from build123d import *

# Parameters (mm, degrees)
F0_W     = 23
F0_H     = 10
F1_DEPTH = 4
F3_DEPTH = 10.001
F4_W     = 19
F4_H     = 6
F5_DEPTH = 8.001
F6_W     = 6
F6_H     = 4
F8_W     = 2.8015887365
F8_H     = 1.9735014066
F11_R    = 1


# Not quite as in the source:
# - a feature of the source that left no trace in its solid (it failed there, or was rolled back) is left out


with BuildPart() as f1:
    # F0 (on Front) → F1 (new body, symmetric)
    with BuildSketch(Plane.XZ):
        Rectangle(F0_W, F0_H)
    extrude(amount=F1_DEPTH, both=True)

    # F2 (on face) → F3 (cut, through all)
    with BuildSketch(Plane.XY.offset(5)):
        with BuildLine():
            ThreePointArc((-6.62e-08, -4), (-5.9424321941, -3.2376566126), (-11.5, -1))
            Line((-11.5, -1), (-11.5, -4))
            Line((-11.5, -4), (-6.62e-08, -4))
        make_face()
        with BuildLine():
            ThreePointArc((11.5, -1), (5.94243213, -3.2376566294), (-6.62e-08, -4))
            Line((-6.62e-08, -4), (11.5, -4))
            Line((11.5, -4), (11.5, -1))
        make_face()
    extrude(amount=-F3_DEPTH, mode=Mode.SUBTRACT)

    # F4 (on face) → F5 (cut, through all)
    with BuildSketch(Plane(origin=(0, 4, 0), x_dir=(-1, 0, 0), z_dir=(0, 1, 0))):
        Rectangle(F4_W, F4_H)
    extrude(amount=-F5_DEPTH, mode=Mode.SUBTRACT)

    # F6 (on face) → F9 section 0
    with BuildSketch(Plane(origin=(0, 0, 3), x_dir=(1, 0, 0), z_dir=(0, 0, -1))):
        Rectangle(F6_W, F6_H)
    # F8 (on offset) → F9 section 1
    with BuildSketch(Plane(origin=(0, 0, 1), x_dir=(1, 0, 0), z_dir=(0, 0, -1))):
        Rectangle(F8_W, F8_H)
    loft()

    # F11
    f11_edges = [f1.edges().sort_by_distance(p)[0] for p in [
        (11.5, 1.5, -5),
        (-11.5, 1.5, -5),
        (11.5, 1.5, 5),
        (-11.5, 1.5, 5),
        (11.5, -1, 0),
        (11.5, 4, 0),
        (0, 4, -5),
        (0, -4, -5),
        (0, -4, 5),
        (-11.5, -1, 0),
        (0, 4, 5),
        (-11.5, 4, 0),
    ]]
    fillet(f11_edges, radius=F11_R)


solid = f1.part
For this review, take the finished solid that the model builds, in its own axes (mm). A direction names the side the tool comes from. Round coordinates to 2 decimals unless told otherwise and drop trailing zeros. Loops run counter-clockwise (first coordinate to the right, second up) from the corner with the lowest first, then second, coordinate; pieces in that order, holes last. Notation, with made-up numbers: (12.25, 0) - (67.25, 0) arc R18 cw to (67.25, 9) - close; hole circle Ø9 at (-34, -32.75). An arc over 180 degrees is marked (long way). One line per item, written item: value. Start each with the question number.
Item 1: The part is to be moulded in two halves that separate along Z. For faces 3 (the flat face through (9.5, 1, 0)), 4 (the cylindrical face through (0.147, 3.699, -4.715)), 5 (the cylindrical face through (-11.215, 1.321, 4.699)), say which applies: +Z half, -Z half, draft (parallel to the pull), parting line (faces both ways), or undercut.
Item 2: Take a section at A-A (z = -0.25). Give the boundary of the cut face in (x, y).
Item 3: Take a section at C-C (z = 4.25). Give the boundary of the cut face in (x, y).
Item 4: For faces 1 (the cylindrical face through (11.199, 1.274, -4.715)), 2 (the flat face through (0, 0, -3)), list the 3-axis set-ups (+Z, -Z, +X, -X, +Y, -Y) from which the entire face can be reached by the end or side of a thin tool; tool diameter is ignored.
Item 5: For L1, parallel to Z at x = -7.75, y = 1.25; L2, parallel to X at y = 2, z = -1.5; L3, parallel to X at y = -1, z = 0.5, list the stretches that pass through material, from the lowest coordinate up.
Item 6: Take a section at B-B (z = 3.25). Give the boundary of the cut face in (x, y).
Answer below:
1. face 3: undercut
1. face 4: -Z half
1. face 5: +Z half
2. outline: (-11.5, -0.41) arc R1 ccw to (-10.97, -1.29) arc R23.54 ccw to (-9.5, -2) - (-9.5, 4) - (-10.5, 4) arc R1 ccw to (-11.5, 3) - close; (9.5, -2) arc R23.54 ccw to (10.97, -1.29) arc R1 ccw to (11.5, -0.41) - (11.5, 3) arc R1 ccw to (10.5, 4) - (9.5, 4) - close
3. outline: (-11.47, -0.41) arc R0.97 ccw to (-10.95, -1.26) arc R23.51 ccw to (10.95, -1.26) arc R0.97 ccw to (11.47, -0.41) - (11.47, 3) arc R0.97 ccw to (10.5, 3.97) - (-10.5, 3.97) arc R0.97 ccw to (-11.47, 3) - close
4. face 1: -Z, +X, +Y, -Y
4. face 2: +Y, -Y
5. L1: z = -5 to -3, 3 to 5
5. L2: x = -11.5 to -9.5, 9.5 to 11.5
5. L3: x = -11.3 to -9.5, 9.5 to 11.3
6. outline: (-11.5, -0.41) arc R1 ccw to (-10.97, -1.29) arc R23.54 ccw to (10.97, -1.29) arc R1 ccw to (11.5, -0.41) - (11.5, 3) arc R1 ccw to (10.5, 4) - (-10.5, 4) arc R1 ccw to (-11.5, 3) - close
